Design review of the part built by this model. Coordinates are the model's own, in mm. Face numbers are marked on the shaded views. Coordinates: 2 decimals unless noted, no trailing zeros. Loops run counter-clockwise (first coordinate to the right, second up) from the corner with the lowest first, then second, coordinate; pieces in that order, holes last.
Q1. Add section B-B on y = 152. Give the boundary of the cut face in (x, z), and give its area (3 significant figures).
Q2. Wall thickness on probe 1 along Z at (x, y) = (-57, 218); probe 2 along X at (y, z) = (426, -293); probe 3 along Y at (x, z) = (-344, -585): over which ranges is each line inside the solid? List them lowest first.
Q3. Add section D-D on y = 5.5. Give the boundary of the cut face in (x, z).
Q4. Draft analysis for pull direction X (two halves, no side actions). For the marked faces 1 and 2, state which applies: released by +X, released by -X, zero draft, split by the parting line, or undercut.
Q5. For P1, Ø16, axis at x = 371.5, z = 86.5, coming from the +Y side; P2, Ø6, axis at x = 387.5, z = 88.5, coming from the -Y side; P3, Ø24, axis at x = 389, z = -478.5, coming from the -Y side; P4, Ø8, axis at x = -317.5, z = -334.5, coming from the +Y side, all flat-tipped, find the tip position at first contact; note any pin that passes through.
Q6. Add section A-A on z = -540. Give the boundary of the cut face in (x, y).
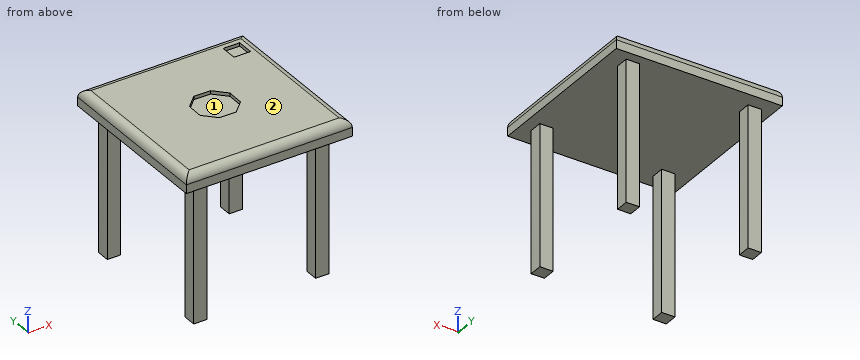
```python
from build123d import *

# Parameters (mm, degrees)
F0_W     = 1000
F0_H     = 1000
F1_DEPTH = 100
F2_R     = 48.284271
F4_DEPTH = 20
F5_W     = 100
F5_H     = 100
F6_DEPTH = 20
F7_W     = 80
F7_H     = 80
F8_DEPTH = 850


with BuildPart() as f1:
    # F0 (on Top) → F1 (new body)
    with BuildSketch(Plane.XY):
        Rectangle(F0_W, F0_H)
    extrude(amount=F1_DEPTH)

    # F2
    f2_edges = [f1.edges().sort_by_distance(p)[0] for p in [
        (0, 500, 100),
        (-500, 0, 100),
        (0, -500, 100),
        (500, 0, 100),
    ]]
    fillet(f2_edges, radius=F2_R)

    # F3 (on face) → F4 (cut)
    with BuildSketch(Plane.XY.offset(100)):
        Polygon((-47.904409, 121.557539), (-119.827693, 52.080628), (-121.557539, -47.904409), (-52.080628, -119.827693), (47.904409, -121.557539), (119.827693, -52.080628), (121.557539, 47.904409), (52.080628, 119.827693), align=None)
    extrude(amount=-F4_DEPTH, mode=Mode.SUBTRACT)

    # F5 (on face) → F6 (cut)
    with BuildSketch(Plane.XY.offset(100)):
        with Locations((375.25773, 372.018505)):
            Rectangle(F5_W, F5_H)
    extrude(amount=-F6_DEPTH, mode=Mode.SUBTRACT)

    # F7 (on face) → F8 (join)
    with BuildSketch(Plane(origin=(0, 0, 0), x_dir=(1, 0, 0), z_dir=(0, 0, -1))):
        with Locations((-362.403053, 378.894394)):
            Rectangle(F7_W, F7_H)
        with Locations((390.322966, 350.974482)):
            Rectangle(F7_W, F7_H)
        with Locations((362.403053, -401.751537)):
            Rectangle(F7_W, F7_H)
        with Locations((-390.322966, -373.831624)):
            Rectangle(F7_W, F7_H)
    extrude(amount=F8_DEPTH)


solid = f1.part
```
Entries:
1. outline: (-500, 0) - (500, 0) - (500, 51.72) arc R48.28 ccw to (451.72, 100) - (-451.72, 100) arc R48.28 ccw to (-500, 51.72) - close
1. area: 99,000 mm2
2. probe 1: z = 0 to 100
2. probe 2: x = 322.4 to 402.4
2. probe 3: y = -418.89 to -338.89
3. outline: (-500, 0) - (500, 0) - (500, 51.72) arc R48.28 ccw to (451.72, 100) - (120.82, 100) - (120.82, 80) - (-120.63, 80) - (-120.63, 100) - (-451.72, 100) arc R48.28 ccw to (-500, 51.72) - close
4. face 1: undercut
4. face 2: zero draft
5. P1: stops at y = 491.89
5. P2: stops at y = -486.21
5. P3: stops at y = -390.97
5. P4: passes through
6. outline: (-430.32, 333.83) - (-350.32, 333.83) - (-350.32, 413.83) - (-430.32, 413.83) - close; (-402.4, -418.89) - (-322.4, -418.89) - (-322.4, -338.89) - (-402.4, -338.89) - close; (322.4, 361.75) - (402.4, 361.75) - (402.4, 441.75) - (322.4, 441.75) - close; (350.32, -390.97) - (430.32, -390.97) - (430.32, -310.97) - (350.32, -310.97) - close
